```python
from build123d import *

# Parameters (mm, degrees)
SKETCH1_R           = 19.05
BOSS_EXTRUDE1_DEPTH = 5
CHAMFER1_SIZE       = 1.905
CHAMFER1_SIZE2      = 1.099852263
SKETCH2_R           = 1
CUT_EXTRUDE1_DEPTH  = 30
SKETCH5_R           = 17.15
CUT_EXTRUDE2_DEPTH  = 15


with BuildPart() as part:
    # Sketch1 → Boss-Extrude1 (new body)
    with BuildSketch(Plane.XY):
        Circle(SKETCH1_R)
    extrude(amount=BOSS_EXTRUDE1_DEPTH)

    # Chamfer1
    chamfer1_edges = [part.edges().sort_by_distance(p)[0] for p in [
        (-19.05, 0, 5),
    ]]
    chamfer1_side = [part.faces().sort_by_distance(p)[0] for p in [
        (-19.05, 0, 2.5),
    ]]
    chamfer(chamfer1_edges, length=CHAMFER1_SIZE, length2=CHAMFER1_SIZE2, reference=chamfer1_side[0])

    # Sketch4 → Revolve-Thin1 (revolve)
    with BuildSketch(Plane.XY.offset(2)):
        Polygon((0, 0), (-12, 20.784609691), (-12.866025404, 20.284609691), (-0.866025404, -0.5), align=None)
    revolve(axis=Axis((0, 0, 2), (-0.5, 0.866025404, 0)))

    # Sketch2 → Cut-Extrude1 (cut)
    with BuildSketch(Plane(origin=(0, 0, 0), x_dir=(1, 0, 0), z_dir=(0, 1, 0))):
        with Locations((0, -2)):
            Circle(SKETCH2_R)
    extrude(amount=CUT_EXTRUDE1_DEPTH, mode=Mode.SUBTRACT)

    # Sketch5 → Cut-Extrude2 (cut)
    with BuildSketch(Plane.XY.offset(5)):
        Circle(SKETCH5_R)
    extrude(amount=-CUT_EXTRUDE2_DEPTH, mode=Mode.SUBTRACT)


solid = part.part
```
Source: CAD feature listing. Evaluate the final solid. Frame: model axes, mm. A direction names the side the tool comes from. Round coordinates to 2 decimals unless told otherwise and drop trailing zeros. Order: outer loops, then holes, each group sorted by start corner. A loop starts at its lowest first (then second) coordinate and runs counter-clockwise, first axis right, second up. Notation, with made-up numbers: (-1.5, 41.25) -> (57.5, 41.25) arc R17 ccw to (57.5, 50.25) -> close; hole circle Ø3 at (61, 53). An arc over 180 degrees is marked (long way). One line per item, written item: value. Start each with the question number.
Q1. Access query for faces 4 (the cylindrical face through (0, 18, 3)), 5 (the flat face through (-16, 7, 0)). Directions: +Z, -Z, +X, -X, +Y, -Y. A direction counts if a zero-diameter tool reaches every point of the face in a straight line with its end or side. Return the directions, or none.
Q2. Pin query (flat end, axial travel): pin 1 (1.5 mm diameter, centred on x = -11.5, z = 4, fed in from -Y); pin 2 (2 mm diameter, centred on y = 8, z = 3.5, fed in from +X); pin 3 (1.2 mm diameter, centred on x = 0, z = 2, fed in from -Y); pin 4 (20.5 mm diameter, centred on x = 0, y = 0, fed in from -Z). Return the tip coordinate at first contact, or that it passes through.
Q3. Section query A-A (y = 0). Return the cut outline in (x, z) (3 decimals), plus the area to 3 significant figures.
Q4. Draft query along X for faces 1 (the flat face through (-12.01, 20.78, 2.01)), 2 (the cylindrical face through (-10.1, 18.968, 2.676)), 3 (the flat face through (15, -9, 5)). Return one class per face: pulls with the +X half, pulls with the -X half, needs draft (parallel to the pull), parting line crosses it, or undercut.
Q5. Material intervals for probe 1 along Y at (x, z) = (0, 2.65); probe 2 along Z at (x, y) = (0, 18.2); probe 3 along Y at (x, z) = (-1.5, 0.45), sorted ascending.
Q6. Section query C-C (z = 2). Return the cut outline in (x, y), plus the area to 3 significant figures.
Q7. Section query B-B (x = 0). Return the cut outline in (y, z) (3 decimals), plus the area to 3 significant figures.
Findings below:
1. face 4: +Y
1. face 5: -Z, +X, -X, +Y, -Y
2. pin 1: y = -15.31
2. pin 2: x = 17.68
2. pin 3: y = -19.05
2. pin 4: through
3. outline: (-19.05, 0) -> (-17.15, 0) -> (-17.15, 5) -> (-17.95, 5) -> (-19.05, 3.095) -> close; (17.15, 0) -> (19.05, 0) -> (19.05, 3.095) -> (17.95, 5) -> (17.15, 5) -> close
3. area: 16.9 mm²
4. face 1: pulls with the -X half
4. face 2: undercut
4. face 3: needs draft
5. probe 1: -19.05 to -17.15
5. probe 2: 0 to 1, 3 to 4.57
5. probe 3: -18.99 to -17.08, 17.08 to 18.99
6. outline: (-12.87, 20.28) -> (-10.38, 15.98) arc R19.05 ccw (long way) to (1, 19.02) -> (1, 17.12) arc R17.15 cw (long way) to (-1, 17.12) -> (-1, 19.02) arc R19.05 ccw to (-8.65, 16.98) -> (-11.13, 21.28) -> close
6. area: 222 mm²
7. outline: (-19.05, 0) -> (-17.15, 0) -> (-17.15, 5) -> (-17.95, 5) -> (-19.05, 3.095) -> close; (17.15, 0) -> (19.05, 0) -> (19.05, 1) -> (17.15, 1) -> close; (17.15, 3) -> (19.05, 3) -> (19.05, 3.095) -> (17.95, 5) -> (17.15, 5) -> close
7. area: 13.1 mm²
